Answer from the drawing. Dimensions are ordinates in mm from the lowest x, y and z of the part. A direction names the side the tool comes from. Give positions to 0.01 mm unless a question says otherwise; leave off trailing zeros. Loops run counter-clockwise (first coordinate to the right, second up) from the corner with the lowest first, then second, coordinate; pieces in that order, holes last. Notation, with made-up numbers: (7.5, 40.5) - (11.5, 40.5) arc R12 ccw to (11.5, 59.5) - close; hole circle Ø11 at (-27, 62). An arc over 180 degrees is marked (long way). Put each result on its own line as item: value. Start each with the question number.
1. A cutting plane is placed at D-D, the plane x = 6. Determine the outline of the cut face in (y, z), plus the area to 3 significant figures.
2. Consider L1, parallel to Y at x = 36, z = 1.2; L2, parallel to X at y = 38.5, z = 2.8; L3, parallel to Y at x = 25, z = 3.25. Determine where each line is inside the solid, lowest interval first. Write a range as from..to.
3. Given pin 1 Ø2 at (y, z) = (7, 4) entering from -X; pin 2 Ø2.5 at (x, z) = (63, 2) entering from +Y; pin 3 Ø2 at (y, z) = (31.5, 0.5) entering from +X, each flat-ended and moving along its own axis, determine where each tip first touches the part or whether it passes through.
4. For the marked faces 1, 2 and 3, determine the directions among +Z, -Z, +X, -X, +Y, -Y from which every point of the face is accessible in a straight line to the end or side of a thin tool.
5. A cutting plane is placed at A-A, the plane x = 36. Determine the outline of the cut face in (y, z), plus the area to 3 significant figures.
6. A cutting plane is placed at B-B, the plane z = 3.85. Determine the outline of the cut face in (x, y), plus the area to 3 significant figures.
7. A cutting plane is placed at C-C, the plane y = 20.5. Determine the outline of the cut face in (x, z).
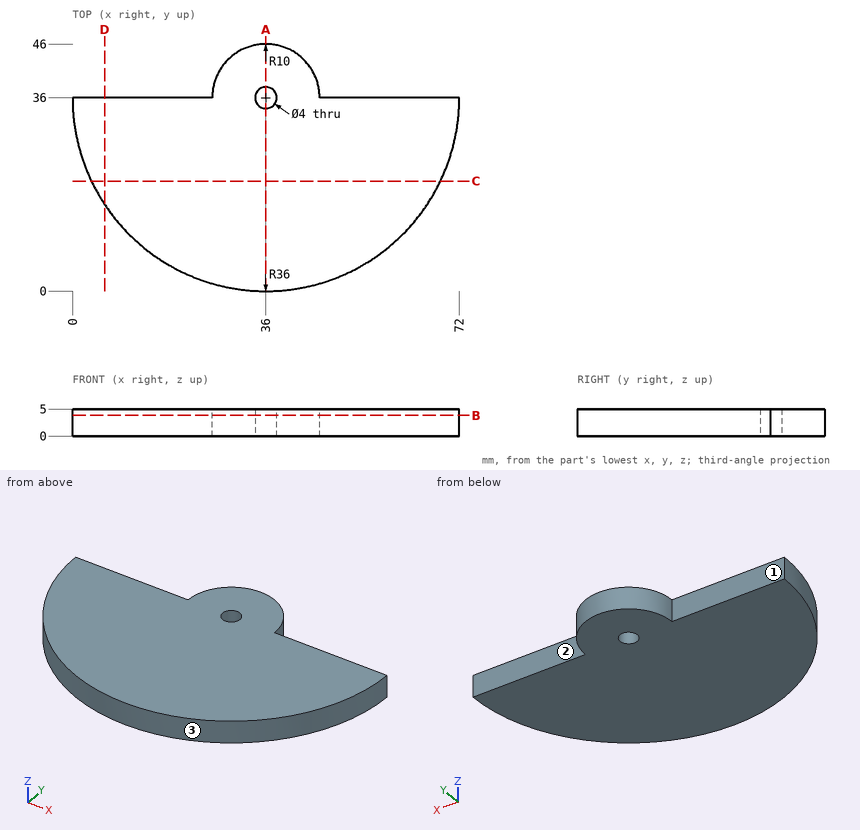
Return value:
1. outline: (16.1, 0) - (36, 0) - (36, 5) - (16.1, 5) - close
1. area: 99.5 mm2
2. L1: y = 0..34, 38..46
2. L2: x = 26.32..45.68
2. L3: y = 1.72..36
3. pin 1: stops at x = 13.37
3. pin 2: stops at y = 36
3. pin 3: stops at x = 71.83
4. face 1: +Z, -Z, -X, +Y
4. face 2: +Z, -Z, +X, +Y
4. face 3: +Z, -Z, -Y
5. outline: (0, 0) - (34, 0) - (34, 5) - (0, 5) - close; (38, 0) - (46, 0) - (46, 5) - (38, 5) - close
5. area: 210 mm2
6. outline: (0, 36) arc R36 ccw to (72, 36) - (46, 36) arc R10 ccw to (26, 36) - close; hole circle Ø4 at (36, 36)
6. area: 2,180 mm2
7. outline: (3.51, 0) - (68.49, 0) - (68.49, 5) - (3.51, 5) - close
